For this review, take the finished solid that the model builds, in its own axes (mm). A direction names the side the tool comes from. Give positions to 0.01 mm unless a question says otherwise; leave off trailing zeros. Order: outer loops, then holes, each group sorted by start corner. A loop starts at its lowest first (then second) coordinate and runs counter-clockwise, first axis right, second up. Notation, with made-up numbers: M -15,-1.75 L -11,-1.75 A20 cw -11,37.25 Z; hole C 26.25,-31.5 d10. An arc over 180 degrees is marked long. Answer as CSV lines item,"result". Start each with the question number.
1. For line 1 along Z through (x, y) = (-0.5, -2.4); line 2 along X through (y, z) = (-0.6, -3); line 3 along Z through (x, y) = (-13.5, -0.75), list the stretches that pass through material, from the lowest coordinate up.
2. We need section D-D, the plane x = -37. Give the boundary of the cut face in (y, z), and give its area (3 significant figures).
3. Clearance check with flat-ended pins moving along their axes: P1, Ø1, axis at y = -2.5, z = 20.5, coming from the +X side; P2, Ø2.5, axis at x = 0, z = -37, coming from the -Y side (3 decimals); P3, Ø6.5, axis at x = 26.163, z = 26.163, coming from the +Y side; P4, Ø1.5, axis at x = 2.5, z = 19, coming from the -Y side. State where each tip first meets the part, or that it passes through.
4. We need section A-A, the plane z = 0. State how many separate pieces and enclosed holes the cut face has, and give its area (3 significant figures).
5. Machinability: for faces 1 (the cylindrical face through (-24.497, -2.442, 24.885)), 2 (the cylindrical face through (-23.977, -2.507, 1.055)), which of the approach directions +Z, -Z, +X, -X, +Y, -Y give a long, thin tool a straight path to every point of the face, cutting with its end or side? Answer none if there is none.
6. Mouldability with a two-part tool opening along Z and no side actions: class faces 3 (the flat face through (0, -2, 20)), 4 (the flat face through (19, -3, -18)) as pulls with the +Z half, pulls with the -Z half, needs draft (parallel to the pull), parting line crosses it, or undercut.
7. We need section C-C, the plane z = -37. Give the boundary of the cut face in (x, y), and give its area (3 significant figures).
Autodesk Inventor part; units mm, degrees
ref_plane "YZ Plane" through (0, 0, 0) normal (1, 0, 0) x (0, 1, 0)
ref_plane "XZ Plane" through (0, 0, 0) normal (0, 1, 0) x (-1, 0, 0)
ref_plane "XY Plane" through (0, 0, 0) normal (0, 0, 1) x (1, 0, 0)
sketch "Sketch1" plane through (0, 0, 0) normal (0, 1, 0) x (-1, 0, 0)
  circle A0 centre (0, 0) radius 42
  circle A1 centre (0, 0) radius 19.5
  circle A2 centre (0, -37) radius 2.1
  circle A3 centre (26.163, -26.163) radius 2.1
  circle A4 centre (37, 0) radius 2.1
  circle A5 centre (26.163, 26.163) radius 2.1
  circle A6 centre (0, 37) radius 2.1
  circle A7 centre (-26.163, 26.163) radius 2.1
  circle A8 centre (-37, 0) radius 2.1
  circle A9 centre (-26.163, -26.163) radius 2.1
  dimension "d0" = 84
  dimension "d1" = 39
  dimension "d2" = 4.2
  dimension "d3" = 37
  dimension "d6" = 360
extrude "Extrusion1" add sketch "Sketch1" against normal blind 3
sketch "Sketch2" plane through (0, -3, 0) normal (0, -1, 0) x (1, 0, 0)
  circle A0 centre (0, 0) radius 24
  dimension "d10" = 48
extrude "Extrusion2" cut sketch "Sketch2" against normal blind 1
hole "Hole1" at (37, 0, 0) at (26.163, 0, 26.163) at (0, 0, 37) at (-26.163, 0, 26.163) at (-37, 0, 0) at (-26.163, 0, -26.163) at (0, 0, -37) at (26.163, 0, -26.163) direction (0, -1, 0) diameter 4.2 end through all countersink diameter 8 countersink angle 90
sketch "Sketch3" plane through (0, 0, 0) normal (0, 1, 0) x (1, 0, 0)
  circle A0 centre (-4.8621, -27.5746) radius 1.5
  circle A1 centre (4.8621, -27.5746) radius 1.5
  circle A2 centre (14, -24.2487) radius 1.5
  circle A3 centre (21.4492, -17.9981) radius 1.5
  circle A4 centre (26.3114, -9.5766) radius 1.5
  circle A5 centre (28, 0) radius 1.5
  circle A6 centre (26.3114, 9.5766) radius 1.5
  circle A7 centre (21.4492, 17.9981) radius 1.5
  circle A8 centre (14, 24.2487) radius 1.5
  circle A9 centre (4.8621, 27.5746) radius 1.5
  circle A10 centre (-4.8621, 27.5746) radius 1.5
  circle A11 centre (-14, 24.2487) radius 1.5
  circle A12 centre (-21.4492, 17.9981) radius 1.5
  circle A13 centre (-26.3114, 9.5766) radius 1.5
  circle A14 centre (-28, 0) radius 1.5
  circle A15 centre (-26.3114, -9.5766) radius 1.5
  circle A16 centre (-21.4492, -17.9981) radius 1.5
  circle A17 centre (-14, -24.2487) radius 1.5
  line L0 (0, 0) -> (-4.8621, -27.5746) construction
  line L1 (0, 0) -> (0, -11.0753) construction
  dimension "d20" = 3
  dimension "d21" = 28
  dimension "d24" = 360
  dimension "d64" = 10
extrude "Extrusion3" cut sketch "Sketch3" against normal through all
properties part number "HousingLid" material "Aluminum 6061"
Result set:
1,line 1,"-42 to -39.04, -34.96 to -23.99, 23.99 to 34.96, 39.04 to 42"
1,line 2,"-41.89 to -38.6, -35.4 to -19.27, 19.27 to 35.4, 38.6 to 41.89"
1,line 3,"-39.77 to -25.66, -22.83 to -14.07, 14.07 to 22.83, 25.66 to 39.77"
2,outline,"M -3,-19.87 L 0,-19.87 L 0,-4 L -1.9,-2.1 L -3,-2.1 Z; M -3,2.1 L -1.9,2.1 L 0,4 L 0,19.87 L -3,19.87 Z"
2,area,"103 mm2"
3,P1,"x = 36.93"
3,P2,"through"
3,P3,"y = -0.75"
3,P4,"y = -2"
4,separate pieces,"6"
4,enclosed holes,"0"
4,area,"75.6 mm2"
5,face 1,"+Y, -Y"
5,face 2,"-Y"
6,face 3,"undercut"
6,face 4,"needs draft"
7,outline,"M -19.87,-3 L -2.1,-3 L -2.1,-1.9 L -4,0 L -19.87,0 Z; M 2.1,-3 L 19.87,-3 L 19.87,0 L 4,0 L 2.1,-1.9 Z"
7,area,"103 mm2"
